Geometry: final body of the model. Coordinates: model frame, mm. A direction names the side the tool comes from. Give positions to 0.01 mm unless a question says otherwise; leave off trailing zeros. Write each loop counter-clockwise with the first axis right and the second up, starting at its lowest first coordinate (ties: lowest second). Pieces come first, ordered by that corner, then holes. Notation, with made-up numbers: M -15,85.25 L 15,85.25 A11 ccw 15,96.25 Z; hole C 78,27.25 d7. An arc over 180 degrees is marked long. Use one line per item in the form item = value. Start each with the question number.
Item 1: Section query A-A on x = -40. Return loops of the section in (y, z) (3 decimals).
Item 2: Material intervals for line 1 along X through (y, z) = (24, -4.1) (3 decimals); line 2 along Y through (x, z) = (49, -2.5) (3 decimals), sorted ascending. Write a range as from..to.
Item 3: Pull-direction query (Y, two-part tool) for faces 1 (the flat face through (-73.025, -27, -2)), 2 (the flat face through (-22, 50.8, -2)), 3 (the flat face through (32.657, -49, -2)), 4 (the flat face through (-22, -50.8, -2)); classes: released by +Y, released by -Y, zero draft, split by the parting line, or undercut.
Item 4: Section query B-B on y = 30. Return loops of the section in (x, z) (3 decimals).
Item 5: Access query for faces 5 (the flat face through (-75, -18.266, -2)), 6 (the flat face through (-10.886, -49, -2)), 7 (the flat face through (75, 16.267, -2)). Directions: +Z, -Z, +X, -X, +Y, -Y. A direction counts if a zero-diameter tool reaches every point of the face in a straight line with its end or side. Return the directions, or none.
Item 6: Contact query for flat-ended pins moving along their axis: P1, Ø2, axis at x = -45, y = 26, coming from the +Z side; P2, Ø2, axis at x = 48, z = -1.5, coming from the -Y side (3 decimals). Output: stop coordinate, or through.
from build123d import *

# Parameters (mm, degrees)
F0_W     = 3.175
F0_H     = 14.0914226329
F0_H_2   = 17.2664226329
F0_H_3   = 12.0928868353
F0_W_2   = 18.5964285714
F0_H_4   = 3.175
F0_W_3   = 21.7714285714
F1_DEPTH = 4.29735


with BuildPart() as f1:
    # F0 (on Top) → F1 (new body)
    with BuildSketch(Plane.XY):
        with Locations((74.6125, 40.5792886835)):
            Rectangle(F0_W, F0_H)
        with Locations((74.6125, 7.6339434177)):
            Rectangle(F0_W, F0_H_2)
        with Locations((74.6125, -9.6324792153)):
            Rectangle(F0_W, F0_H_2)
        with Locations((74.6125, -41.5785565823)):
            Rectangle(F0_W, F0_H_3)
        with Locations((63.7267857143, -49.2125)):
            Rectangle(F0_W_2, F0_H_4)
        with Locations((21.7714285714, -49.2125)):
            Rectangle(F0_W_3, F0_H_4)
        with Locations((-21.7714285714, -49.2125)):
            Rectangle(F0_W_3, F0_H_4)
        with Locations((-63.7267857143, -49.2125)):
            Rectangle(F0_W_2, F0_H_4)
        with Locations((-74.6125, -41.5785565823)):
            Rectangle(F0_W, F0_H_3)
        with Locations((-74.6125, -9.6324792153)):
            Rectangle(F0_W, F0_H_2)
        with Locations((-74.6125, 7.6339434177)):
            Rectangle(F0_W, F0_H_2)
        with Locations((-74.6125, 40.5792886835)):
            Rectangle(F0_W, F0_H)
        with Locations((-63.7267857143, 49.2125)):
            Rectangle(F0_W_2, F0_H_4)
        with Locations((-21.7714285714, 49.2125)):
            Rectangle(F0_W_3, F0_H_4)
        with Locations((21.7714285714, 49.2125)):
            Rectangle(F0_W_3, F0_H_4)
        with Locations((63.7267857143, 49.2125)):
            Rectangle(F0_W_2, F0_H_4)
        Polygon((54.4285714286, -47.625), (73.025, -47.625), (73.025, -35.5321131647), (73.025, -18.2656905317), (73.025, -0.9992678988), (73.025, 16.2671547341), (73.025, 33.5335773671), (73.025, 47.625), (54.4285714286, 47.625), (32.6571428571, 47.625), (10.8857142857, 47.625), (-10.8857142857, 47.625), (-32.6571428571, 47.625), (-54.4285714286, 47.625), (-73.025, 47.625), (-73.025, 33.5335773671), (-73.025, 16.2671547341), (-73.025, -0.9992678988), (-73.025, -18.2656905317), (-73.025, -35.5321131647), (-73.025, -47.625), (-54.4285714286, -47.625), (-32.6571428571, -47.625), (-10.8857142857, -47.625), (10.8857142857, -47.625), (32.6571428571, -47.625), align=None)
        with Locations((74.6125, 49.2125)):
            Rectangle(F0_W, F0_H_4)
        with Locations((74.6125, -49.2125)):
            Rectangle(F0_W, F0_H_4)
        with Locations((-74.6125, -49.2125)):
            Rectangle(F0_W, F0_H_4)
        with Locations((-74.6125, 49.2125)):
            Rectangle(F0_W, F0_H_4)
    extrude(amount=-F1_DEPTH)


solid = f1.part
Answer sheet:
q1.outline = M -47.625,-4.297 L 47.625,-4.297 L 47.625,0 L -47.625,0 Z
q2.line_1 = -73.025..73.025
q2.line_2 = -47.625..47.625
q3.face_1 = undercut
q3.face_2 = released by +Y
q3.face_3 = zero draft
q3.face_4 = released by -Y
q4.outline = M -73.025,-4.297 L 73.025,-4.297 L 73.025,0 L -73.025,0 Z
q5.face_5 = +Z, -Z, -X
q5.face_6 = +Z, -Z, -Y
q5.face_7 = +Z, -Z, +X
q6.P1 = 0
q6.P2 = -47.625
